The listing builds one solid part. Answer for the finished solid, in the listing's coordinates (mm). A direction names the side the tool comes from. Give positions to 0.01 mm unless a question says otherwise; leave off trailing zeros. Write each loop counter-clockwise with the first axis right and the second up, starting at its lowest first coordinate (ties: lowest second). Pieces come first, ordered by that corner, then holes. Notation, with made-up numbers: (79.5, 49.25) - (101.5, 49.25) arc R36 ccw to (101.5, 83.25) - close; hole circle Ø8 at (-14, 13.25). An arc over 180 degrees is marked (long way). Return JSON: item names as keys, results as strings.
from build123d import *

# Parameters (mm, degrees)
SKETCH_1_W          = 40
SKETCH_1_H          = 40
EXTRUDE_1_DEPTH     = 17
SKETCH_2_W          = 39
SKETCH_2_H          = 39
EXTRUDE_2_DEPTH     = 11
SKETCH_3_W          = 2
SKETCH_3_H          = 39
CUT_EXTRUDE_1_DEPTH = 9
EXTRUDE_3_DEPTH     = 11
SKETCH_5_R          = 5.444681892
EXTRUDE_4_DEPTH     = 11
SKETCH_6_W          = 25
SKETCH_6_H          = 17.382728094
EXTRUDE_5_DEPTH     = 11
SKETCH_7_R          = 4.5
EXTRUDE_6_DEPTH     = 11
EXTRUDE_6_TAPER     = 17
SKETCH_8_W          = 17
SKETCH_8_H          = 10.324195756
EXTRUDE_7_DEPTH     = 11
SKETCH_9_R          = 8.784415214
CUT_EXTRUDE_2_DEPTH = 27
CUT_EXTRUDE_START   = 10
SKETCH_10_W         = 58.477636184
SKETCH_10_H         = 70.793077964
CUT_EXTRUDE_3_DEPTH = 47
SKETCH_11_W         = 62.750592471
SKETCH_11_H         = 80.218393182
CUT_EXTRUDE_4_DEPTH = 22


with BuildPart() as part:
    # Эскиз1 → Бобышка-Вытянуть1 (new body)
    with BuildSketch(Plane(origin=(0, 0, 0), x_dir=(0, 0, -1), z_dir=(1, 0, 0))):
        Rectangle(SKETCH_1_W, SKETCH_1_H)
    extrude(amount=EXTRUDE_1_DEPTH)

    # Эскиз2 → Бобышка-Вытянуть2 (add)
    with BuildSketch(Plane(origin=(17, 0, 0), x_dir=(0, 0, -1), z_dir=(1, 0, 0))):
        Rectangle(SKETCH_2_W, SKETCH_2_H)
    extrude(amount=EXTRUDE_2_DEPTH)

    # Эскиз3 → Вырез-Вытянуть1 (cut)
    with BuildSketch(Plane(origin=(28, 0, 0), x_dir=(0, 0, -1), z_dir=(1, 0, 0))):
        with Locations((-16, 0)):
            Rectangle(SKETCH_3_W, SKETCH_3_H)
        with Locations((-12, 0)):
            Rectangle(SKETCH_3_W, SKETCH_3_H)
        with Locations((-8, 0)):
            Rectangle(SKETCH_3_W, SKETCH_3_H)
        with Locations((-4, 0)):
            Rectangle(SKETCH_3_W, SKETCH_3_H)
        Rectangle(SKETCH_3_W, SKETCH_3_H)
        with Locations((4, 0)):
            Rectangle(SKETCH_3_W, SKETCH_3_H)
        with Locations((8, 0)):
            Rectangle(SKETCH_3_W, SKETCH_3_H)
        with Locations((12, 0)):
            Rectangle(SKETCH_3_W, SKETCH_3_H)
        with Locations((16, 0)):
            Rectangle(SKETCH_3_W, SKETCH_3_H)
    extrude(amount=-CUT_EXTRUDE_1_DEPTH, mode=Mode.SUBTRACT)

    # Эскиз4 → Бобышка-Вытянуть3 (add)
    with BuildSketch(Plane(origin=(28, 0, 0), x_dir=(0, 0, -1), z_dir=(1, 0, 0))):
        with BuildLine():
            Line((13.94108797, 18.534083609), (-13.965803425, 18.534083609))
            ThreePointArc((-13.965803425, 18.534083609), (-17.501337331, 17.069617515), (-18.965803425, 13.534083609))
            Line((-18.965803425, 13.534083609), (-18.965803425, -13.794341936))
            ThreePointArc((-18.965803425, -13.794341936), (-17.501337331, -17.329875842), (-13.965803425, -18.794341936))
            Line((-13.965803425, -18.794341936), (13.94108797, -18.794341936))
            ThreePointArc((13.94108797, -18.794341936), (17.476621876, -17.329875842), (18.94108797, -13.794341936))
            Line((18.94108797, -13.794341936), (18.94108797, 13.534083609))
            ThreePointArc((18.94108797, 13.534083609), (17.476621876, 17.069617515), (13.94108797, 18.534083609))
        make_face()
    extrude(amount=EXTRUDE_3_DEPTH)

    # Эскиз5 → Бобышка-Вытянуть4 (add)
    with BuildSketch(Plane.XZ.offset(20)):
        with Locations(Location((7.767128211, 5.128320155, 0), (0, 0, 90))):
            Circle(SKETCH_5_R)
    extrude(amount=EXTRUDE_4_DEPTH)

    # Эскиз6 → Бобышка-Вытянуть5 (add)
    with BuildSketch(Plane.XZ.offset(31)):
        with Locations((10.668319864, 5.154067921)):
            Rectangle(SKETCH_6_W, SKETCH_6_H)
    extrude(amount=EXTRUDE_5_DEPTH)

    # Эскиз7 → Бобышка-Вытянуть6 (add)
    with BuildSketch(Plane.XZ.offset(42)):
        with Locations((7.710138854, 5.107455984)):
            Circle(SKETCH_7_R)
    extrude(amount=EXTRUDE_6_DEPTH, taper=EXTRUDE_6_TAPER)

    # Эскиз8 → Бобышка-Вытянуть7 (add)
    with BuildSketch(Plane(origin=(0, 0, -20), x_dir=(-1, 0, 0), z_dir=(0, 0, -1))):
        with Locations((-8.5, 14.837902122)):
            Rectangle(SKETCH_8_W, SKETCH_8_H)
    extrude(amount=EXTRUDE_7_DEPTH)

    # Эскиз9 → Вырез-Вытянуть2 (cut)
    with BuildSketch(Plane(origin=(17, 0, 0), x_dir=(0, 0, -1), z_dir=(1, 0, 0))):
        with Locations((31, 20)):
            Circle(SKETCH_9_R)
    extrude(amount=-CUT_EXTRUDE_2_DEPTH, mode=Mode.SUBTRACT)

    # Эскиз10 → Вырез-Вытянуть3 (cut)
    with BuildSketch(Plane.XZ.offset(20).offset(CUT_EXTRUDE_START)):
        with Locations((4.776161953, -4.159448177)):
            Rectangle(SKETCH_10_W, SKETCH_10_H)
    extrude(amount=CUT_EXTRUDE_3_DEPTH, mode=Mode.SUBTRACT)

    # Эскиз11 → Вырез-Вытянуть4 (cut)
    with BuildSketch(Plane(origin=(39, 0, 0), x_dir=(0, 0, -1), z_dir=(1, 0, 0))):
        with Locations((5.568785854, 6.666933577)):
            Rectangle(SKETCH_11_W, SKETCH_11_H)
    extrude(amount=-CUT_EXTRUDE_4_DEPTH, mode=Mode.SUBTRACT)


solid = part.part
Item 1: A cutting plane is placed at A-A on x = 14.75. Determine the outline of the cut face in (y, z), then the cut area to 3 significant figures.
Answer below:
{"outline": "(-20, -20) - (9.68, -20) - (9.68, -31) - (11.22, -31) arc R8.78 cw to (20, -22.22) - (20, 20) - (-20, 20) - close", "area": "1,650 mm²"}
Item 2: Consider L1, parallel to Y at x = 3.5, z = -2; L2, parallel to Z at x = 8.75, y = -25. Determine where each line is inside the solid, lowest interval first.
Answer below:
{"L1": "y = -20 to 20", "L2": "z = -0.23 to 10.48"}
Item 3: For faces 1 (the face through (2.37, -24.93, 4.42)), 2 (the face through (9, 10, -31)), 3 (the face through (9, 9.676, -25)), determine the directions among +Z, -Z, +X, -X, +Y, -Y from which every point of the face is accessible in a straight line to the end or side of a thin tool.
Answer below:
{"face 1": "-Y", "face 2": "-Z, +X, -X, +Y, -Y", "face 3": "-Z, +X, -X, -Y"}
Item 4: Flat-ended cylindrical pins translate along their axes: P1, Ø8, axis at x = 3.5, z = -6.5, coming from the -Y side; P2, Ø1, axis at y = 9, z = -26, coming from the -X side; P3, Ø1.5, axis at x = 14, y = -8.5, coming from the -Z side; P4, Ø5.5, axis at x = 11.5, z = -24, coming from the -Y side. Find the tip coordinate at first contact, or state that the pin passes through.
Answer below:
{"P1": "stops at y = -20", "P2": "passes through", "P3": "stops at z = -20", "P4": "stops at y = 9.68"}
Item 5: A cutting plane is placed at C-C on y = -12.5. Determine the outline of the cut face in (x, z).
Answer below:
{"outline": "(0, -20) - (17, -20) - (17, 20) - (0, 20) - close"}
Item 6: A cutting plane is placed at B-B on z = 0.5. Determine the outline of the cut face in (x, y).
Answer below:
{"outline": "(0, -20) - (4.9, -20) - (4.9, -30) - (10.63, -30) - (10.63, -20) - (17, -20) - (17, 20) - (0, 20) - close"}
Item 7: A cutting plane is placed at D-D on x = 5.5. Determine the outline of the cut face in (y, z).
Answer below:
{"outline": "(-30, 0.18) - (-20, 0.18) - (-20, -20) - (9.68, -20) - (9.68, -31) - (11.22, -31) arc R8.78 cw to (20, -22.22) - (20, 20) - (-20, 20) - (-20, 10.08) - (-30, 10.08) - close"}
